Here's the drawing with two shaded views (mm, measured from the low corner). I have some questions. A direction names the side the tool comes from. Coordinates: 2 decimals unless noted, no trailing zeros. Write each loop counter-clockwise with the first axis right and the second up, starting at its lowest first coordinate (ties: lowest second). Pieces come first, ordered by that corner, then holes. Notation, with made-up numbers: (33.5, 12) -> (91.5, 12) arc R21 ccw to (91.5, 18) -> close; hole circle Ø10 at (54.5, 27). An arc over 180 degrees is marked (long way). Answer in a Markdown table with one row per item. Add a question column.
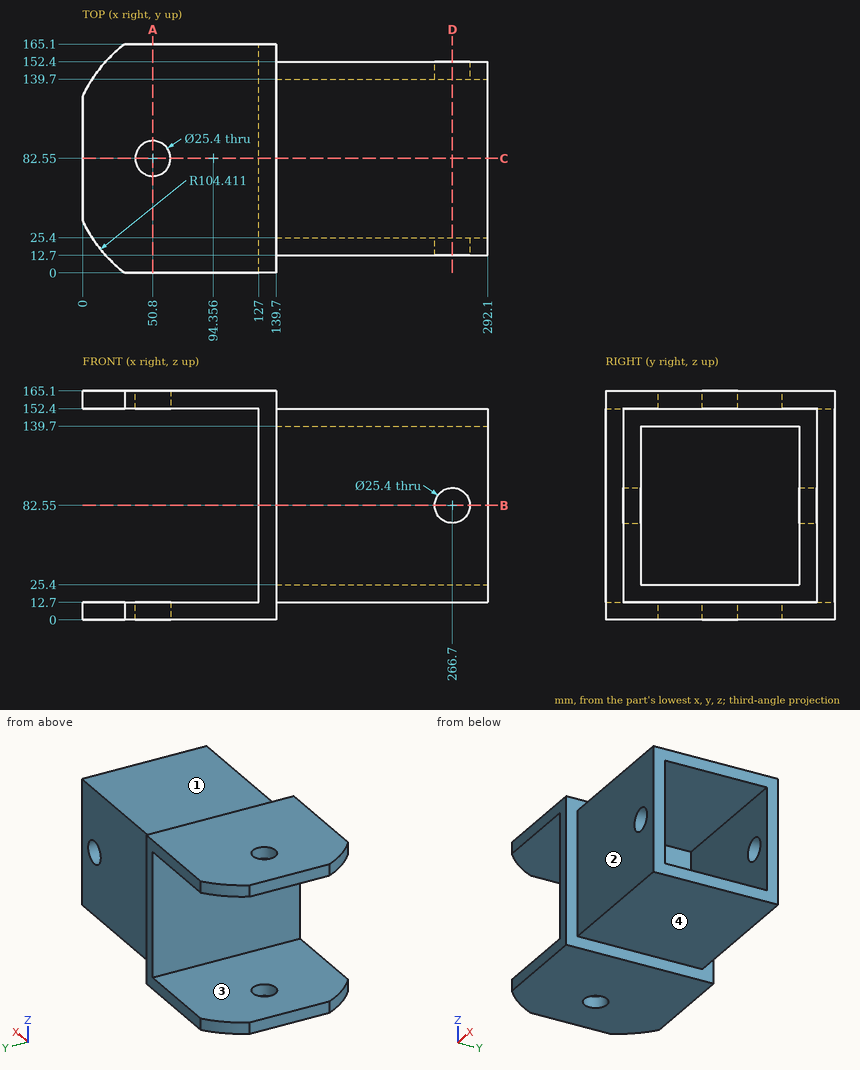
Q1. For the marked faces 1, 2, 3 and 4, which set-ups out of +Z, -Z, +X, -X, +Y, -Y let a thin tool reach every point of the face, with its end or its side?
Q2. Imagine slicing it at A-A on x = 50.8. Please give me the cut outline in (y, z).
Q3. Imagine slicing it at C-C on y = 82.55. Please give me the cut outline in (x, z), plus the area to 3 significant figures.
Q4. Imagine slicing it at D-D on x = 266.7. Please give me the cut outline in (y, z).
Q5. Imagine slicing it at B-B on z = 82.55. Please give me the cut outline in (x, y).
Q6. I need wall thicknesses on line 1 (Y direction, x = 50.8, z = 161); line 2 (Z direction, x = 100, y = 114); line 3 (Z direction, x = 266.7, y = 144.25). Which ranges of each line are inside material? Lowest first, please. Write a range as [from, to].
Q7. I'm going to push flat-ended pins straight in: P1, Ø1.5, axis at y = 81, z = 80.5, coming from the -X side; P2, Ø1, axis at x = 152.5, z = 114.5, coming from the +Y side; P3, Ø3, axis at x = 161, y = 52.5, coming from the +Z side. Where does each tip first touch, or does it pass through?
Result sheet:
| question | item | result |
|---|---|---|
| 1 | face 1 | +Z, +X, +Y, -Y |
| 1 | face 2 | +Z, -Z, +X, -Y |
| 1 | face 3 | -X, +Y, -Y |
| 1 | face 4 | -Z, +X, +Y, -Y |
| 2 | outline | (0, 0) -> (69.85, 0) -> (69.85, 12.7) -> (0, 12.7) -> close; (0, 152.4) -> (69.85, 152.4) -> (69.85, 165.1) -> (0, 165.1) -> close; (95.25, 0) -> (165.1, 0) -> (165.1, 12.7) -> (95.25, 12.7) -> close; (95.25, 152.4) -> (165.1, 152.4) -> (165.1, 165.1) -> (95.25, 165.1) -> close |
| 3 | outline | (0, 0) -> (38.1, 0) -> (38.1, 12.7) -> (0, 12.7) -> close; (0, 152.4) -> (38.1, 152.4) -> (38.1, 165.1) -> (0, 165.1) -> close; (63.5, 0) -> (139.7, 0) -> (139.7, 12.7) -> (292.1, 12.7) -> (292.1, 25.4) -> (139.7, 25.4) -> (139.7, 139.7) -> (292.1, 139.7) -> (292.1, 152.4) -> (139.7, 152.4) -> (139.7, 165.1) -> (63.5, 165.1) -> (63.5, 152.4) -> (127, 152.4) -> (127, 12.7) -> (63.5, 12.7) -> close |
| 3 | area | 8,550 mm^2 |
| 4 | outline | (12.7, 12.7) -> (152.4, 12.7) -> (152.4, 69.85) -> (139.7, 69.85) -> (139.7, 25.4) -> (25.4, 25.4) -> (25.4, 69.85) -> (12.7, 69.85) -> close; (12.7, 95.25) -> (25.4, 95.25) -> (25.4, 139.7) -> (139.7, 139.7) -> (139.7, 95.25) -> (152.4, 95.25) -> (152.4, 152.4) -> (12.7, 152.4) -> close |
| 5 | outline | (127, 0) -> (139.7, 0) -> (139.7, 12.7) -> (254, 12.7) -> (254, 25.4) -> (139.7, 25.4) -> (139.7, 139.7) -> (254, 139.7) -> (254, 152.4) -> (139.7, 152.4) -> (139.7, 165.1) -> (127, 165.1) -> close; (279.4, 12.7) -> (292.1, 12.7) -> (292.1, 25.4) -> (279.4, 25.4) -> close; (279.4, 139.7) -> (292.1, 139.7) -> (292.1, 152.4) -> (279.4, 152.4) -> close |
| 6 | line 1 | y = [0, 69.85], [95.25, 165.1] |
| 6 | line 2 | z = [0, 12.7], [152.4, 165.1] |
| 6 | line 3 | z = [12.7, 69.85], [95.25, 152.4] |
| 7 | P1 | stops at x = 127 |
| 7 | P2 | stops at y = 152.4 |
| 7 | P3 | stops at z = 152.4 |
